from build123d import *

# Parameters (mm, degrees)
SKETCH1_W                 = 40
SKETCH1_H                 = 21
BOSS_EXTRUDE1_DEPTH       = 150
CUT_EXTRUDE1_DEPTH        = 152.691298366
CUT_EXTRUDE1_DEPTH_BACK   = 152.691298366
SKETCH2_W                 = 4
SKETCH2_H                 = 6.5
M4X0_7_TAPPED_HOLE1_D     = 3.3
M4X0_7_TAPPED_HOLE1_DEPTH = 10.1
M4X0_7_TAPPED_HOLE1_TIP   = 0.991420021
M4X0_7_TAPPED_HOLE2_D     = 3.3
M4X0_7_TAPPED_HOLE2_DEPTH = 10.1
M4X0_7_TAPPED_HOLE2_TIP   = 0.991420021


with BuildPart() as part:
    # Sketch1 → Boss-Extrude1 (new, symmetric)
    with BuildSketch(Plane.XY):
        Rectangle(SKETCH1_W, SKETCH1_H)
    extrude(amount=BOSS_EXTRUDE1_DEPTH, both=True)

    # Sketch2 → Cut-Extrude1 (cut, two sides: drawn at the far end of the back side and taken through both)
    with BuildSketch(Plane.XY.offset(-CUT_EXTRUDE1_DEPTH_BACK)):
        with Locations((9.9, 7.25)):
            Rectangle(SKETCH2_W, SKETCH2_H)
        with Locations((-9.9, 7.25)):
            Rectangle(SKETCH2_W, SKETCH2_H)
        with Locations((9.9, -7.25)):
            Rectangle(SKETCH2_W, SKETCH2_H)
        with Locations((-9.9, -7.25)):
            Rectangle(SKETCH2_W, SKETCH2_H)
    extrude(amount=CUT_EXTRUDE1_DEPTH + CUT_EXTRUDE1_DEPTH_BACK, mode=Mode.SUBTRACT)

    # M4x0.7 Tapped Hole1
    with Locations(Plane.XY.offset(150)):
        with Locations((-12, -0.5), (12, -0.5)):
            Hole(M4X0_7_TAPPED_HOLE1_D / 2, depth=M4X0_7_TAPPED_HOLE1_DEPTH)
            with Locations((0, 0, -(M4X0_7_TAPPED_HOLE1_DEPTH + M4X0_7_TAPPED_HOLE1_TIP / 2))):  # 118° drill point
                Cone(0, M4X0_7_TAPPED_HOLE1_D / 2, M4X0_7_TAPPED_HOLE1_TIP, mode=Mode.SUBTRACT)

    # M4x0.7 Tapped Hole2
    with Locations(Plane(origin=(0, 0, -150), x_dir=(-1, 0, 0), z_dir=(0, 0, -1))):
        with Locations((-12, -0.5), (12, -0.5)):
            Hole(M4X0_7_TAPPED_HOLE2_D / 2, depth=M4X0_7_TAPPED_HOLE2_DEPTH)
            with Locations((0, 0, -(M4X0_7_TAPPED_HOLE2_DEPTH + M4X0_7_TAPPED_HOLE2_TIP / 2))):  # 118° drill point
                Cone(0, M4X0_7_TAPPED_HOLE2_D / 2, M4X0_7_TAPPED_HOLE2_TIP, mode=Mode.SUBTRACT)


solid = part.part
Can you work these out from the model? Positions are in its coordinate system, mm. A direction names the side the tool comes from. Round coordinates to 2 decimals unless told otherwise and drop trailing zeros. Write each loop counter-clockwise with the first axis right and the second up, starting at its lowest first coordinate (ties: lowest second). Pieces come first, ordered by that corner, then holes. Notation, with made-up numbers: (41.25, 29) -> (76.25, 29) arc R16 cw to (76.25, 57) -> close; hole circle Ø2 at (44.25, 38.5). An arc over 180 degrees is marked (long way). Use one line per item in the form item = value. Start each with the question number.
Q1. I'm going to push flat-ended pins straight in: P1, Ø4.5, axis at x = 9, z = -21.5, coming from the -Y side; P2, Ø2, axis at x = -10.5, z = 22.5, coming from the -Y side; P3, Ø2.5, axis at x = -12, y = -0.5, coming from the +Z side; P4, Ø2, axis at x = 10, z = -18, coming from the +Y side. Where does each tip first touch, or does it pass through?
Q2. Imagine slicing it at B-B (z = -98). Please give me the cut outline in (x, y), then the cut area to 3 significant figures.
Q3. We'd pull the mould along X, two halves only. Please class faces 4 (the face through (16, -10.5, 2)), 5 (the face through (-20, 0, 2)), 6 (the face through (11.9, 7, -2)), 7 (the face through (7.9, 7, -2)): +X half, -X half, draft (parallel to the pull), parting line (faces both ways), or undercut.
Q4. Imagine slicing it at A-A (y = -7.25). Please give me the cut outline in (x, z).
Q5. If I drill on probe 1 along X at (y, z) = (5.5, 61); probe 2 along X at (y, z) = (-0.5, -144); probe 3 along Y at (x, z) = (12, -146.5), over which ranges is the centre line in solid material (lowest first)? Write a range as [from, to].
Q6. Which directions (+Z, -Z, +X, -X, +Y, -Y) give clear straight access to the entire face, cutting with the end or side of a thin tool? Please do faces 1 (the face through (-7.9, 7, -2)), 2 (the face through (7.9, -7, -2)), 3 (the face through (-16, -10.5, 2)).
Worked out:
q1.P1 = -10.5
q1.P2 = -4
q1.P3 = 139.66
q1.P4 = 4
q2.outline = (-20, -10.5) -> (-11.9, -10.5) -> (-11.9, -4) -> (-7.9, -4) -> (-7.9, -10.5) -> (7.9, -10.5) -> (7.9, -4) -> (11.9, -4) -> (11.9, -10.5) -> (20, -10.5) -> (20, 10.5) -> (11.9, 10.5) -> (11.9, 4) -> (7.9, 4) -> (7.9, 10.5) -> (-7.9, 10.5) -> (-7.9, 4) -> (-11.9, 4) -> (-11.9, 10.5) -> (-20, 10.5) -> close
q2.area = 736 mm^2
q3.face_4 = draft
q3.face_5 = -X half
q3.face_6 = undercut
q3.face_7 = undercut
q4.outline = (-20, -150) -> (-11.9, -150) -> (-11.9, 150) -> (-20, 150) -> close; (-7.9, -150) -> (7.9, -150) -> (7.9, 150) -> (-7.9, 150) -> close; (11.9, -150) -> (20, -150) -> (20, 150) -> (11.9, 150) -> close
q5.probe_1 = [-20, -11.9], [-7.9, 7.9], [11.9, 20]
q5.probe_2 = [-20, -13.65], [-10.35, 10.35], [13.65, 20]
q5.probe_3 = [-10.5, -2.15], [1.15, 10.5]
q6.face_1 = +Z, -Z, +Y
q6.face_2 = +Z, -Z, -Y
q6.face_3 = +Z, -Z, +X, -X, -Y
